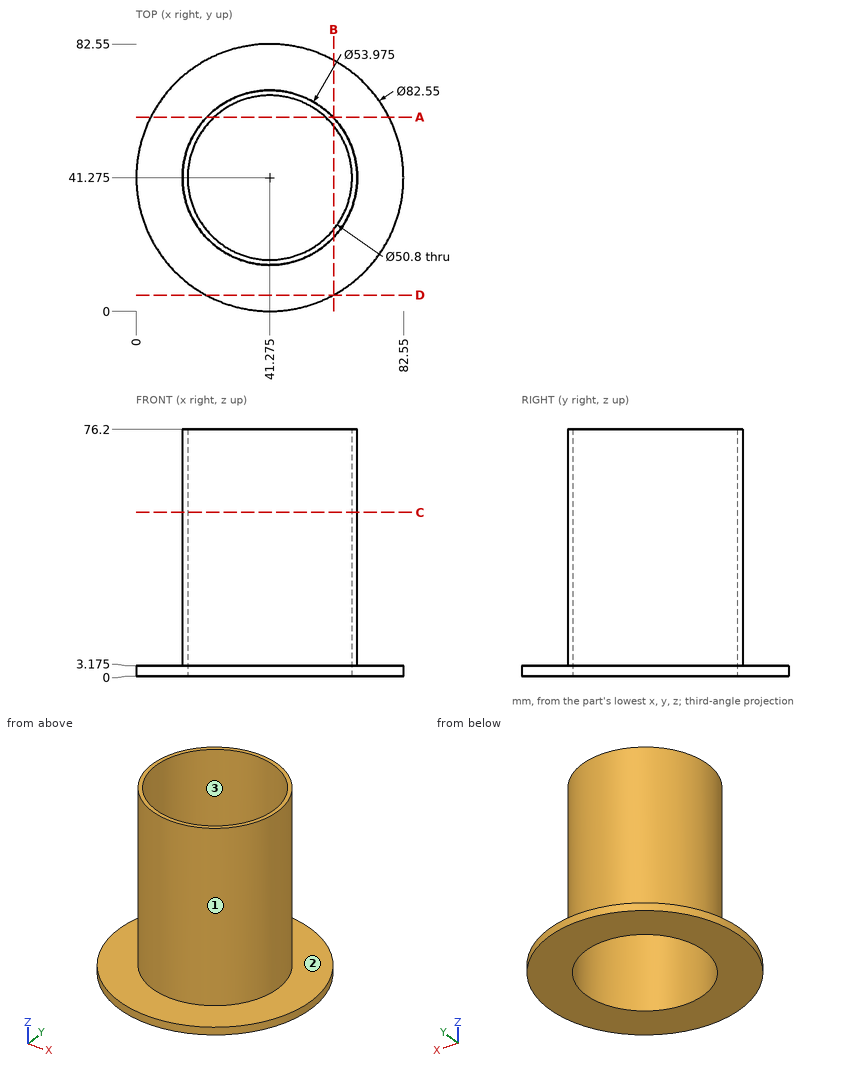
Print and shaded views of the part. All mm, measured from the part's lowest x, y and z. Give positions to 0.01 mm unless a question says otherwise; leave off trailing zeros. Order: outer loops, then holes, each group sorted by start corner. A loop starts at its lowest first (then second) coordinate and runs counter-clockwise, first axis right, second up. Notation, with made-up numbers: M -16,51.25 L 26,51.25 A22 ccw 26,67.25 Z; hole C -27.75,20 d1. An arc over 180 degrees is marked long. Use one line per item in the form item = value.
Q1. Slice it at D-D, the plane y = 5. Write the cut outline in (x, z) (3 decimals), and give its area (3 significant figures).
Conclusion:
outline = M 21.584,0 L 60.966,0 L 60.966,3.175 L 21.584,3.175 Z
area = 125 mm2
Q2. Slice it at A-A, the plane y = 60. Write the cut outline in (x, z) (1 decimal).
Conclusion:
outline = M 4.5,0 L 24.1,0 L 24.1,76.2 L 21.8,76.2 L 21.8,3.2 L 4.5,3.2 Z; M 58.4,0 L 78.1,0 L 78.1,3.2 L 60.7,3.2 L 60.7,76.2 L 58.4,76.2 Z
Q3. Slice it at B-B, the plane x = 61. Write the cut outline in (y, z) (3 decimals), and give its area (3 significant figures).
Conclusion:
outline = M 5.018,0 L 25.272,0 L 25.272,76.2 L 22.856,76.2 L 22.856,3.175 L 5.018,3.175 Z; M 57.278,0 L 77.532,0 L 77.532,3.175 L 59.694,3.175 L 59.694,76.2 L 57.278,76.2 Z
area = 481 mm2
Q4. Slice it at C-C, the plane z = 50.5. Write the cut outline in (x, y) (1 decimal), and give its area (3 significant figures).
Conclusion:
outline = C 41.3,41.3 d54; hole C 41.3,41.3 d50.8
area = 261 mm2
Q5. Pull direction X, two halves, no side cores. Call the marked faces 1, 2 and 3: released by +X, released by -X, zero draft, split by the parting line, or undercut.
Conclusion:
face_1 = split by the parting line
face_2 = zero draft
face_3 = undercut
Q6. Pin check, flat tips, straight feed: P1, Ø1, axis at y = 65.5, z = 31, coming from the -X side; P2, Ø3, axis at y = 58, z = 33, coming from the +X side; P3, Ø4, axis at x = 42, z = 43.5, coming from the +Y side; P4, Ø6, axis at x = 17.5, y = 54.5, coming from the -Z side. Stop position of each tip, or through.
Conclusion:
P1 = 28.41
P2 = 63.56
P3 = 68.26
P4 = 0
Q7. Wall check: probe 1 along Z at (x, y) = (74, 54) (3 decimals); probe 2 along X at (y, z) = (56, 8.5); probe 3 along X at (y, z) = (48, 22). Give the ranges that are in metal, low to high.
Conclusion:
probe_1 = 0 to 3.175
probe_2 = 18.66 to 20.58, 61.97 to 63.89
probe_3 = 15.14 to 16.78, 65.77 to 67.41
